Design review of the part built by this model. Coordinates are the model's own, in mm. A direction names the side the tool comes from. Round coordinates to 2 decimals unless told otherwise and drop trailing zeros. Order: outer loops, then holes, each group sorted by start corner. A loop starts at its lowest first (then second) coordinate and runs counter-clockwise, first axis right, second up.
from build123d import *

# Parameters (mm, degrees)
SKETCH_1_R          = 2.5
EXTRUDE_1_DEPTH     = 15
SKETCH_2_OUTSIDE_W  = 15.65
SKETCH_2_OUTSIDE_H  = 21.15
CUT_EXTRUDE_1_DEPTH = 11.740715169


with BuildPart() as part:
    # 草圖1 → 填料-伸長1 (new body)
    with BuildSketch(Plane.XY):
        with BuildLine():
            Line((3.5, -2.937484093), (5.5, -1.259284831))
            Line((5.5, -1.259284831), (5.5, 6.740715169))
            Line((5.5, 6.740715169), (3.5, 6.740715169))
            Line((3.5, 6.740715169), (3.5, 5.809475019))
            ThreePointArc((3.5, 5.809475019), (2.724744871, 4.228336189), (1, 3.872983346))
            ThreePointArc((1, 3.872983346), (-3.878905774, -0.976775304), (2.714993039, -2.937484093))
            Line((2.714993039, -2.937484093), (3.5, -2.937484093))
        make_face()
        Circle(SKETCH_1_R, mode=Mode.SUBTRACT)
    extrude(amount=EXTRUDE_1_DEPTH)

    # 草圖2 outside → 除料-伸長1 (cut, through all)
    with BuildSketch(Plane(origin=(0, 6.740715169, 0), x_dir=(1, 0, 0), z_dir=(0, 1, 0))):
        with Locations((0.75, -7.5)):
            Rectangle(SKETCH_2_OUTSIDE_W, SKETCH_2_OUTSIDE_H)
        with BuildLine():
            Line((5.5, -15), (3.5, -15))
            ThreePointArc((3.5, -15), (0.571067812, -7.928932188), (-6.5, -5))
            Line((-6.5, -5), (-4, -5))
            Line((-4, -5), (-4, 0))
            Line((-4, 0), (5.5, 0))
            Line((5.5, 0), (5.5, -5))
            ThreePointArc((5.5, -5), (5, -7.5), (5.5, -10))
            Line((5.5, -10), (5.5, -15))
        make_face(mode=Mode.SUBTRACT)
    extrude(amount=-CUT_EXTRUDE_1_DEPTH, mode=Mode.SUBTRACT)


solid = part.part
1) Take a section at A-A on y = 0. Give the boundary of the cut face in (x, z).
Results:
outline: (-4, 0) - (-2.5, 0) - (-2.5, 5.83) arc R10 cw to (-4, 5.32) - close; (2.5, 0) - (5.5, 0) - (5.5, 5) arc R6.5 cw to (5.5, 10) - (5.5, 15) - (3.5, 15) arc R10 cw to (2.5, 10.64) - close
2) To check wall thickness, follow line 1 along Y through (x, z) = (0, 5.75); line 2 along X through (y, z) = (0, 4.5); line 3 along Y through (x, z) = (1.25, 7.5). State the ranges of each line that lie inside material, in increasing order.
Results:
line 1: y = -4 to -2.5, 2.5 to 4
line 2: x = -4 to -2.5, 2.5 to 5.5
line 3: y = -3.8 to -2.17, 2.17 to 3.83
3) Take a section at D-D on z = 13.5. Give the boundary of the cut face in (x, y).
Results:
outline: (3.39, -2.94) - (3.5, -2.94) - (5.5, -1.26) - (5.5, 6.74) - (3.5, 6.74) - (3.5, 5.81) arc R2 cw to (3.39, 5.15) - close
4) The part is to be moulded in two halves that separate along X. For faces 3 (the face through (5.5, 3, 12)), 4 (the face through (2.74, 4.24, 5.73)), 5 (the face through (4, 2, 15)), say which applies: released by +X, released by -X, zero draft, split by the parting line, or undercut.
Results:
face 3: released by +X
face 4: undercut
face 5: zero draft
5) Clearance check with flat-ended pins moving along their axes: P1, Ø1.5, axis at x = 0.5, z = 8.5, coming from the -Y side; P2, Ø6, axis at y = 4.5, z = 8, coming from the -X side; P3, Ø0.5, axis at y = 6, z = 7.5, coming from the -X side. State where each tip first meets the part, or that it passes through.
Results:
P1: stops at y = -3.98
P2: stops at x = -2.99
P3: stops at x = 3.5
6) Take a section at B-B on x = 0. Give the boundary of the cut face in (y, z).
Results:
outline: (-4, 0) - (-2.5, 0) - (-2.5, 7.4) - (-4, 7.4) - close; (2.5, 0) - (4, 0) - (4, 7.4) - (2.5, 7.4) - close
7) Take a section at C-C on z = 1. Give the boundary of the cut face in (x, y) (3 decimals).
Results:
outline: (1, 3.873) arc R4 ccw (long way) to (2.715, -2.937) - (3.5, -2.937) - (5.5, -1.259) - (5.5, 6.741) - (3.5, 6.741) - (3.5, 5.809) arc R2 cw to start; hole circle Ø5 at (0, 0)
8) For faces 1 (the face through (-3.906, -0.864, 3.01)), 2 (the face through (3.5, 6, 7)), list the 3-axis set-ups (+Z, -Z, +X, -X, +Y, -Y) from which the entire face can be reached by the end or side of a thin tool; tool diameter is ignored.
Results:
face 1: +Z, -Z
face 2: +Z, -Z, -X, +Y
